```python
from build123d import *

# Parameters (mm, degrees)
SERVO_SHELF_START                = 21.4
SERVO_SHELF_PROFILE_W            = 46
SERVO_SHELF_PROFILE_H            = 36
SERVO_SHELF_DEPTH                = 4
REAR_CLAMPING_BLOCK_START        = -18
REAR_CLAMPING_BLOCK_PROFILE_W    = 7
REAR_CLAMPING_BLOCK_PROFILE_H    = 10
REAR_CLAMPING_BLOCK_DEPTH        = 36
SERVO_BODY_WINDOW_START          = 20.4
SERVO_BODY_WINDOW_PROFILE_W      = 23.8
SERVO_BODY_WINDOW_PROFILE_H      = 13
SERVO_BODY_WINDOW_DEPTH          = 25.744213361
YAW_SERVO_M2_FASTENERS_START     = 20.4
YAW_SERVO_M2_FASTENERS_PROFILE_R = 1.3
YAW_SERVO_M2_FASTENERS_DEPTH     = 25.744213361
LEFT_NUT_ACCESS_START            = 20
LEFT_NUT_ACCESS_PROFILE_W        = 10
LEFT_NUT_ACCESS_PROFILE_H        = 8
LEFT_NUT_ACCESS_DEPTH            = 26.144213361
RIGHT_NUT_ACCESS_START           = 20
RIGHT_NUT_ACCESS_PROFILE_W       = 10
RIGHT_NUT_ACCESS_PROFILE_H       = 8
RIGHT_NUT_ACCESS_DEPTH           = 26.144213361
REAR_CLAMPING_M3_HOLES_START     = -25
REAR_CLAMPING_M3_PROFILE_R       = 1.6
REAR_CLAMPING_M3_HOLES_DEPTH     = 11


with BuildPart() as part:
    # Servo_shelf_profile → Servo_shelf (new body)
    with BuildSketch(Plane(origin=(0, 0, 0), x_dir=(1, 0, 0), z_dir=(0, 1, 0)).offset(SERVO_SHELF_START)):
        with Locations((2, 0)):
            Rectangle(SERVO_SHELF_PROFILE_W, SERVO_SHELF_PROFILE_H)
    extrude(amount=SERVO_SHELF_DEPTH)

    # Rear_clamping_block_profile → Rear_clamping_block (add)
    with BuildSketch(Plane.XY.offset(REAR_CLAMPING_BLOCK_START)):
        with Locations((-17.5, 28)):
            Rectangle(REAR_CLAMPING_BLOCK_PROFILE_W, REAR_CLAMPING_BLOCK_PROFILE_H)
    extrude(amount=REAR_CLAMPING_BLOCK_DEPTH)

    # Servo_body_window_profile → Servo_body_window (cut, through all)
    with BuildSketch(Plane(origin=(0, 0, 0), x_dir=(1, 0, 0), z_dir=(0, 1, 0)).offset(SERVO_BODY_WINDOW_START)):
        with Locations((5.5, 0)):
            Rectangle(SERVO_BODY_WINDOW_PROFILE_W, SERVO_BODY_WINDOW_PROFILE_H)
    extrude(amount=SERVO_BODY_WINDOW_DEPTH, mode=Mode.SUBTRACT)

    # Yaw_servo_M2_fasteners_profile → Yaw_servo_M2_fasteners (cut, through all)
    with BuildSketch(Plane(origin=(0, 0, 0), x_dir=(1, 0, 0), z_dir=(0, 1, 0)).offset(YAW_SERVO_M2_FASTENERS_START)):
        with Locations(Location((-9, 0, 0), (0, 0, 90))):
            Circle(YAW_SERVO_M2_FASTENERS_PROFILE_R)
        with Locations(Location((20, 0, 0), (0, 0, 90))):
            Circle(YAW_SERVO_M2_FASTENERS_PROFILE_R)
    extrude(amount=YAW_SERVO_M2_FASTENERS_DEPTH, mode=Mode.SUBTRACT)

    # Left_nut_access_profile → Left_nut_access (cut, through all)
    with BuildSketch(Plane(origin=(0, 0, 0), x_dir=(1, 0, 0), z_dir=(0, 1, 0)).offset(LEFT_NUT_ACCESS_START)):
        with Locations((-9, 12)):
            Rectangle(LEFT_NUT_ACCESS_PROFILE_W, LEFT_NUT_ACCESS_PROFILE_H)
    extrude(amount=LEFT_NUT_ACCESS_DEPTH, mode=Mode.SUBTRACT)

    # Right_nut_access_profile → Right_nut_access (cut, through all)
    with BuildSketch(Plane(origin=(0, 0, 0), x_dir=(1, 0, 0), z_dir=(0, 1, 0)).offset(RIGHT_NUT_ACCESS_START)):
        with Locations((-9, -12)):
            Rectangle(RIGHT_NUT_ACCESS_PROFILE_W, RIGHT_NUT_ACCESS_PROFILE_H)
    extrude(amount=RIGHT_NUT_ACCESS_DEPTH, mode=Mode.SUBTRACT)

    # Rear_clamping_M3_profile → Rear_clamping_M3_holes (cut)
    with BuildSketch(Plane(origin=(0, 0, 0), x_dir=(0, 0, -1), z_dir=(1, 0, 0)).offset(REAR_CLAMPING_M3_HOLES_START)):
        with Locations((12, 28)):
            Circle(REAR_CLAMPING_M3_PROFILE_R)
        with Locations((-12, 28)):
            Circle(REAR_CLAMPING_M3_PROFILE_R)
    extrude(amount=REAR_CLAMPING_M3_HOLES_DEPTH, mode=Mode.SUBTRACT)


solid = part.part
```
The listing builds one solid part. Answer for the finished solid, in the listing's coordinates (mm). A direction names the side the tool comes from. Give positions to 0.01 mm unless a question says otherwise; leave off trailing zeros. Order: outer loops, then holes, each group sorted by start corner. A loop starts at its lowest first (then second) coordinate and runs counter-clockwise, first axis right, second up. Notation, with made-up numbers: (59, 38) -> (107, 38) arc R18 cw to (107, 66) -> close; hole circle Ø10 at (71.5, 63). An arc over 180 degrees is marked (long way). Answer as a JSON object with one key per item and string values. Group by question number.
Item 1: Consider L1, parallel to X at y = 22.8, z = 0; L2, parallel to Z at x = -17.75, y = 28; L3, parallel to X at y = 24.5, z = 6. Determine where each line is inside the solid, lowest interval first. Write a range as from..to.
Item 2: The part is cut by section D-D on z = 0. Write down the section's boundary in (x, y), and give its area (3 significant figures).
Item 3: Flat-ended cylindrical pins translate along their axes: pin 1 (1.5 mm diameter, centred on x = 15.5, z = 14, fed in from +Y); pin 2 (2 mm diameter, centred on x = 20, z = 0, fed in from -Y); pin 3 (5 mm diameter, centred on y = 28.5, z = -12.5, fed in from +X). Find the tip coordinate at first contact, or state that the pin passes through.
Item 4: The part is cut by section A-A on z = -5. Write down the section's boundary in (x, y).
Item 5: A tool of negligible diameter and unlimited length cuts with its end or side. For faces 4 (the flat face through (10, 25.4, -8)), 5 (the cylindrical face through (-17.55, 29.08, 13.18)), 6 (the flat face through (-4, 23, 12)), from which of +Z, -Z, +X, -X, +Y, -Y can it reach the whole face along a straight path? Write none if from no direction.
Item 6: The part is cut by section B-B on x = 20. Write down the section's boundary in (y, z).
Item 7: The part is cut by section C-C on y = 28. Write down the section's boundary in (x, z), and give its area (3 significant figures).
Item 8: Determine the mould class of faces 1 (the flat face through (-21, 27, 0)), 2 (the flat face through (25, 23, 0)), 3 (the flat face through (-4, 23, -12)) for opening direction X: pulls with the +X half, pulls with the -X half, needs draft (parallel to the pull), parting line crosses it, or undercut.
Result set:
{
 "1": {"L1": "-21..-10.3, -7.7..-6.4, 17.4..18.7, 21.3..25", "L2": "-18..-13.6, -10.4..10.4, 13.6..18", "L3": "-21..-6.4, 17.4..25"},
 "2": {"outline": "(-21, 21.4) -> (-10.3, 21.4) -> (-10.3, 25.4) -> (-14, 25.4) -> (-14, 33) -> (-21, 33) -> close; (-7.7, 21.4) -> (-6.4, 21.4) -> (-6.4, 25.4) -> (-7.7, 25.4) -> close; (17.4, 21.4) -> (18.7, 21.4) -> (18.7, 25.4) -> (17.4, 25.4) -> close; (21.3, 21.4) -> (25, 21.4) -> (25, 25.4) -> (21.3, 25.4) -> close", "area": "121 mm²"},
 "3": {"pin 1": "y = 25.4", "pin 2": "through", "pin 3": "x = -14"},
 "4": {"outline": "(-21, 21.4) -> (-6.4, 21.4) -> (-6.4, 25.4) -> (-14, 25.4) -> (-14, 33) -> (-21, 33) -> close; (17.4, 21.4) -> (25, 21.4) -> (25, 25.4) -> (17.4, 25.4) -> close"},
 "5": {"face 4": "+Z, -Z, +X, +Y", "face 5": "+X, -X", "face 6": "+Y, -Y"},
 "6": {"outline": "(21.4, -18) -> (25.4, -18) -> (25.4, -1.3) -> (21.4, -1.3) -> close; (21.4, 1.3) -> (25.4, 1.3) -> (25.4, 18) -> (21.4, 18) -> close"},
 "7": {"outline": "(-21, -18) -> (-14, -18) -> (-14, -13.6) -> (-21, -13.6) -> close; (-21, -10.4) -> (-14, -10.4) -> (-14, 10.4) -> (-21, 10.4) -> close; (-21, 13.6) -> (-14, 13.6) -> (-14, 18) -> (-21, 18) -> close", "area": "207 mm²"},
 "8": {"face 1": "pulls with the -X half", "face 2": "pulls with the +X half", "face 3": "undercut"}
}
